Part model, mm, in its own coordinate system. Coordinates: 2 decimals unless noted, no trailing zeros. Loops run counter-clockwise (first coordinate to the right, second up) from the corner with the lowest first, then second, coordinate; pieces in that order, holes last. Notation, with made-up numbers: M -35,77 L -26,77 A7 ccw -26,81 Z; hole C 88.5,4.25 d2. An arc over 180 degrees is marked long. Answer as a JSON object with one key per item and string values. Group by question number.
1. Saw through at A-A on z = 56. Write the cut outline in (x, y).
2. Drill centre lines: L1, parallel to Y at x = 0, z = 101.75; L2, parallel to X at y = 2, z = 97.5; L3, parallel to Z at x = -0.5, y = 1.25. Where is each one in solid material? Low to high.
3. Drop flat-ended pins along their axis: pin 1 Ø3 at (x, y) = (0, 0) entering from +Z; pin 2 Ø2.5 at (x, y) = (0, 0) entering from -Z; pin 3 Ø1.5 at (x, z) = (2, -16) entering from -Y. Give the stop position or say it passes through.
from build123d import *

# Parameters (mm, degrees)
SKETCH_1_R      = 4
EXTRUDE_1_DEPTH = 107
M4X0_71_D       = 3.3
M4X0_71_DEPTH   = 11
M4X0_71_TIP     = 0.991420021
M4X0_72_D       = 3.3
M4X0_72_DEPTH   = 11
M4X0_72_TIP     = 0.991420021


with BuildPart() as part:
    # Эскиз1 → Бобышка-Вытянуть1 (new, symmetric)
    with BuildSketch(Plane.XY):
        Circle(SKETCH_1_R)
    extrude(amount=EXTRUDE_1_DEPTH, both=True)

    # Отверстие обработанное метчиком M4x0.71
    with Locations(Plane(origin=(0, 0, -107), x_dir=(-1, 0, 0), z_dir=(0, 0, -1))):
        with Locations((0, 0)):
            Hole(M4X0_71_D / 2, depth=M4X0_71_DEPTH)
            with Locations((0, 0, -(M4X0_71_DEPTH + M4X0_71_TIP / 2))):  # 118° drill point
                Cone(0, M4X0_71_D / 2, M4X0_71_TIP, mode=Mode.SUBTRACT)

    # Отверстие обработанное метчиком M4x0.72
    with Locations(Plane.XY.offset(107)):
        with Locations((0, 0)):
            Hole(M4X0_72_D / 2, depth=M4X0_72_DEPTH)
            with Locations((0, 0, -(M4X0_72_DEPTH + M4X0_72_TIP / 2))):  # 118° drill point
                Cone(0, M4X0_72_D / 2, M4X0_72_TIP, mode=Mode.SUBTRACT)


solid = part.part
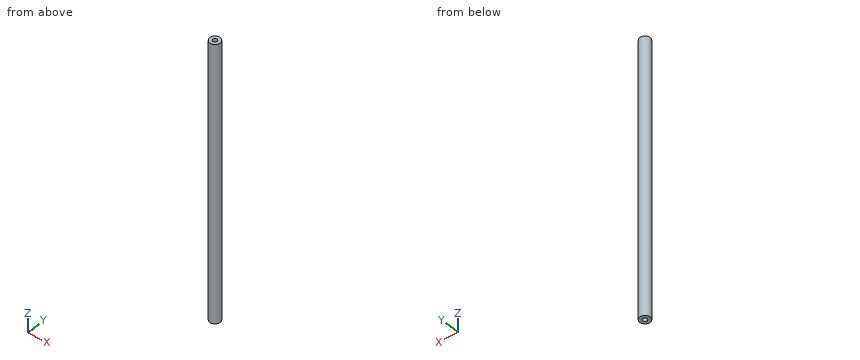
Outcome:
{
 "1": {"outline": "C 0,0 d8"},
 "2": {"L1": "y = -4 to -1.65, 1.65 to 4", "L2": "x = -3.46 to 3.46", "L3": "z = -95.82 to 95.82"},
 "3": {"pin 1": "stops at z = 95.91", "pin 2": "stops at z = -95.76", "pin 3": "stops at y = -3.8"}
}
